```python
from build123d import *

# Parameters (mm, degrees)
SKETCH2_R               = 2.5
CUT_EXTRUDE1_DEPTH      = 7
CUT_EXTRUDE1_DEPTH_BACK = 7
FILLET2_R               = 1
FILLET3_R               = 1
FILLET4_R               = 1.5


with BuildPart() as part:
    # Sketch1 → Revolve1 (revolve)
    with BuildSketch(Plane.XY):
        Polygon((0, 3), (10, 3), (10, 6), (175, 6), (175, 0), (0, 0), align=None)
    revolve(axis=Axis((0, 0, 0), (1, 0, 0)))

    # Sketch2 → Cut-Extrude1 (cut, two sides)
    with BuildSketch(Plane.XY) as cut_extrude1_sk:
        with Locations((5, 0)):
            Circle(SKETCH2_R)
    extrude(amount=CUT_EXTRUDE1_DEPTH, mode=Mode.SUBTRACT)
    extrude(cut_extrude1_sk.sketch, amount=-CUT_EXTRUDE1_DEPTH_BACK, mode=Mode.SUBTRACT)

    # Fillet2
    fillet2_edges = [part.edges().sort_by_distance(p)[0] for p in [
        (0, -3, 0),
    ]]
    fillet(fillet2_edges, radius=FILLET2_R)

    # Fillet3
    fillet3_edges = [part.edges().sort_by_distance(p)[0] for p in [
        (10, -6, 0),
        (10, -3, 0),
    ]]
    fillet(fillet3_edges, radius=FILLET3_R)

    # Fillet4
    fillet4_edges = [part.edges().sort_by_distance(p)[0] for p in [
        (175, -6, 0),
    ]]
    fillet(fillet4_edges, radius=FILLET4_R)


solid = part.part
```
Check sheet for the modelled part. Datum: model origin and axes. Units: mm. Round coordinates to 2 decimals unless told otherwise and drop trailing zeros. Write each loop counter-clockwise with the first axis right and the second up, starting at its lowest first coordinate (ties: lowest second). Pieces come first, ordered by that corner, then holes. Notation, with made-up numbers: (37, 56.25) -> (77, 56.25) arc R25 ccw to (77, 87.25) -> close; hole circle Ø6 at (-14, 48). An arc over 180 degrees is marked (long way). One line per question, with ' | ' between items. Start each with the question number.
1. Sectioned sample at C-C, the plane x = 5. Record the cut outline in (y, z), then the cut area to 3 significant figures.
2. Depth check by flat-ended pin: pin 1 (6.5 mm diameter, centred on x = 5, y = 0, fed in from +Z); pin 2 (1.5 mm diameter, centred on y = 5, z = 0.5, fed in from -X); pin 3 (1 mm diameter, centred on x = 30, z = 4, fed in from -Y). Enter the tip coordinate at first touch or a pass-through.
3. Scan lines: line 1 along X through (y, z) = (0, -0.25); line 2 along X through (y, z) = (4.25, -1.25); line 3 along Y through (x, z) = (108.5, -4.5). Record each from-to range of solid material in increasing order. Write a range as from..to.
4. Release check for a two-part mould opening along X. For faces 1 (the face through (0, 0, 0)), 2 (the face through (175, 0, 0)), 3 (the face through (93, -6, 0)), 4 (the face through (7.385, 0.751, 0.042)) record: +X half, -X half, draft (parallel to the pull), parting line (faces both ways), or undercut.
5. Sectioned sample at B-B, the plane x = 92. Record the cut outline in (y, z), then the cut area to 3 significant figures.
6. Sectioned sample at A-A, the plane z = 0. Record the cut outline in (x, y), then the cut area to 3 significant figures.
Taken from the geometry:
1) outline: (-2.5, -1.66) -> (-2.5, 1.66) arc R3 ccw to start; (2.5, -1.66) arc R3 ccw to (2.5, 1.66) -> close | area: 2.25 mm^2
2) pin 1: stops at z = 3 | pin 2: stops at x = 10 | pin 3: stops at y = -4.87
3) line 1: x = 0..2.5, 7.5..175 | line 2: x = 10..175 | line 3: y = -3.97..3.97
4) face 1: -X half | face 2: +X half | face 3: draft | face 4: undercut
5) outline: circle Ø12 at (0, 0) | area: 113 mm^2
6) outline: (0, -2) arc R1 ccw to (1, -3) -> (9, -3) arc R1 cw to (10, -4) -> (10, -5) arc R1 ccw to (11, -6) -> (173.5, -6) arc R1.5 ccw to (175, -4.5) -> (175, 4.5) arc R1.5 ccw to (173.5, 6) -> (11, 6) arc R1 ccw to (10, 5) -> (10, 4) arc R1 cw to (9, 3) -> (1, 3) arc R1 ccw to (0, 2) -> close; hole circle Ø5 at (5, 0) | area: 2,020 mm^2
